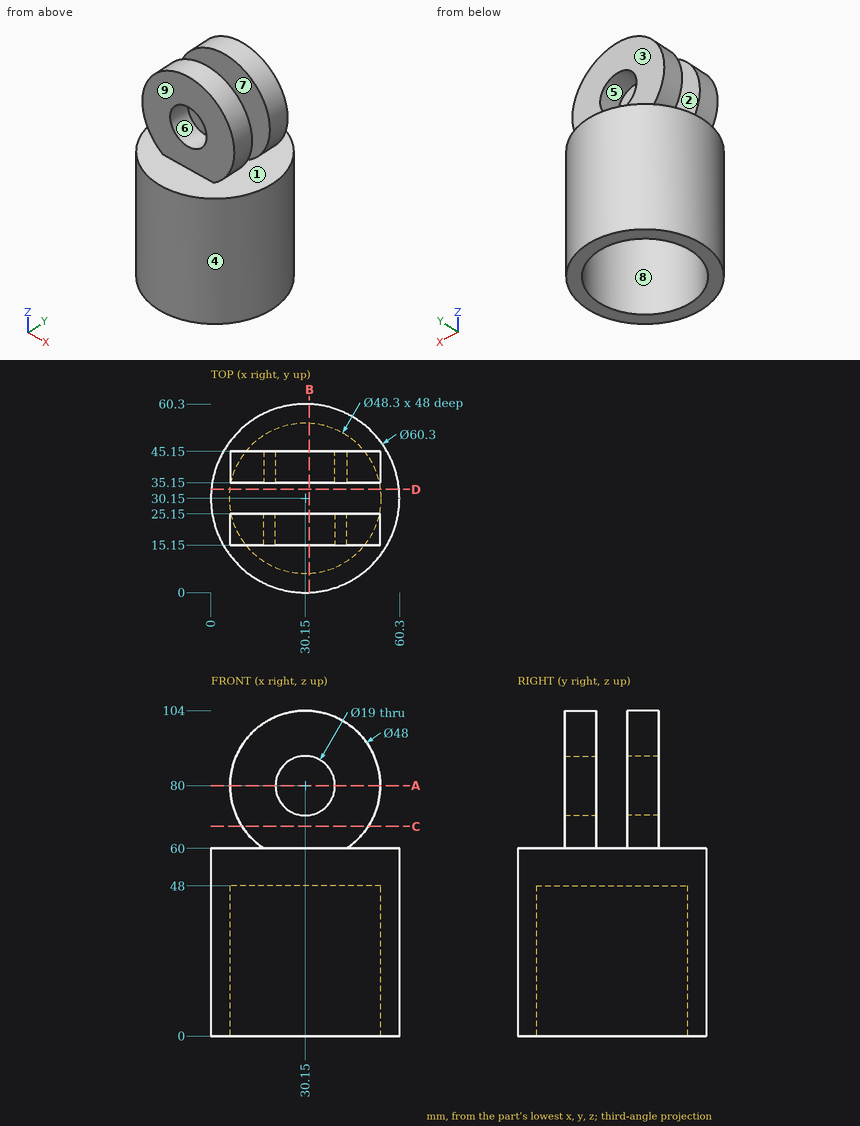
Study the drawing (mm; zero at the part's minimum x, y, z) and answer. A direction names the side the tool comes from. Round coordinates to 2 decimals unless told otherwise and drop trailing zeros. Loops run counter-clockwise (first coordinate to the right, second up) from the corner with the lowest first, then second, coordinate; pieces in that order, holes last. Notation, with made-up numbers: (-22.75, -23) -> (-4.75, -23) arc R7 cw to (-4.75, -15) -> close; hole circle Ø7 at (35.25, 30). An arc over 180 degrees is marked (long way). Write each question's results on one line, items separated by ' | '. Start each with the question number.
1. For a pull along Y with two mould halves and no side action, classify the marked faces 6, 7, 8 and 9 as +Y half, -Y half, draft (parallel to the pull), parting line (faces both ways), or undercut.
2. Section C-C (z = 67) is taken. Determine the outline of the cut face in (x, y).
3. Find the intervals of material crossed by probe 1 along Y at (x, z) = (20, 98); probe 2 along Y at (x, z) = (29.5, 15.5); probe 3 along Z at (x, y) = (30.15, 43), in increasing order. Write a range as from..to.
4. Given pin 1 Ø2 at (x, z) = (54, 92.5) entering from +Y; pin 2 Ø22 at (x, z) = (24, 90) entering from +Y; pin 3 Ø12 at (y, z) = (14.5, 87.5) entering from +X; pin 4 Ø1.5 at (y, z) = (24, 77) entering from +X, each flat-ended and moving along its own axis, determine where each tip first touches the part or whether it passes through.
5. Section B-B (x = 31.5) is taken. Determine the outline of the cut face in (y, z).
6. Section D-D (y = 33) is taken. Determine the outline of the cut face in (x, z) (3 decimals), plus the area to 3 significant figures.
7. A tool of negligible diameter and unlimited length cuts with its end or side. For the marked faces 1, 2, 3, 4 and 5, from which of +Z, -Z, +X, -X, +Y, -Y can it reach the whole face along a straight path? Write none if from no direction.
8. Section A-A (z = 80) is taken. Determine the outline of the cut face in (x, y).
Evaluation:
1) face 6: draft | face 7: undercut | face 8: undercut | face 9: -Y half
2) outline: (9.98, 15.15) -> (50.32, 15.15) -> (50.32, 25.15) -> (9.98, 25.15) -> close; (9.98, 35.15) -> (50.32, 35.15) -> (50.32, 45.15) -> (9.98, 45.15) -> close
3) probe 1: y = 15.15..25.15, 35.15..45.15 | probe 2: y = 0.01..6.01, 54.29..60.29 | probe 3: z = 48..70.5, 89.5..104
4) pin 1: passes through | pin 2: stops at y = 45.15 | pin 3: stops at x = 54.1 | pin 4: stops at x = 54.04
5) outline: (0.03, 0) -> (6.04, 0) -> (6.04, 48) -> (54.26, 48) -> (54.26, 0) -> (60.27, 0) -> (60.27, 60) -> (45.15, 60) -> (45.15, 70.6) -> (35.15, 70.6) -> (35.15, 60) -> (25.15, 60) -> (25.15, 70.6) -> (15.15, 70.6) -> (15.15, 60) -> (0.03, 60) -> close; (15.15, 89.4) -> (25.15, 89.4) -> (25.15, 103.96) -> (15.15, 103.96) -> close; (35.15, 89.4) -> (45.15, 89.4) -> (45.15, 103.96) -> (35.15, 103.96) -> close
6) outline: (0.135, 0) -> (6.169, 0) -> (6.169, 48) -> (54.131, 48) -> (54.131, 0) -> (60.165, 0) -> (60.165, 60) -> (0.135, 60) -> close | area: 1,300 mm2
7) face 1: none | face 2: +Z, +X, -X | face 3: +Z, +X, -X, +Y | face 4: +Z, -Z | face 5: +Y, -Y
8) outline: (6.15, 15.15) -> (20.65, 15.15) -> (20.65, 25.15) -> (6.15, 25.15) -> close; (6.15, 35.15) -> (20.65, 35.15) -> (20.65, 45.15) -> (6.15, 45.15) -> close; (39.65, 15.15) -> (54.15, 15.15) -> (54.15, 25.15) -> (39.65, 25.15) -> close; (39.65, 35.15) -> (54.15, 35.15) -> (54.15, 45.15) -> (39.65, 45.15) -> close
